For this review, take the finished solid that the model builds, in its own axes (mm). A direction names the side the tool comes from. Round coordinates to 2 decimals unless told otherwise and drop trailing zeros. Use a Markdown table: item, result. Add a question column.
1) Draft analysis for pull direction X (two halves, no side actions). For faces 1 (the face through (6.099, 10, -154)), 2 (the face through (26.101, 10, -154)), 3 (the face through (15.7, 15.2, -313)), 4 (the face through (10, 13.901, -154)), state which applies: pulls with the +X half, pulls with the -X half, needs draft (parallel to the pull), parting line crosses it, or undercut.
2) Consider section A-A (z = -151). Give the number of separate pieces and of enclosed holes in the cut face, plus the area to 3 significant figures.
3) Machinability: for faces 5 (the face through (20, 18.2, -154)), 6 (the face through (20, 20, -154)), which of the approach directions +Z, -Z, +X, -X, +Y, -Y give a long, thin tool a straight path to every point of the face, cutting with its end or side? Answer none if there is none.
4) Wall thickness on line 1 along X through (y, z) = (1.75, -137); line 2 along X through (y, z) = (4, -16); line 3 along Y through (x, z) = (34, -42): over which ranges is each line inside the solid? List them lowest first. Write a range as [from, to].
5) Clearance check with flat-ended pins moving along their axes: P1, Ø3, axis at y = 11.5, z = -233.5, coming from the -X side; P2, Ø4.5, axis at y = 10, z = -198.5, coming from the +X side; P3, Ø2, axis at x = 28.5, z = -165.5, coming from the +Y side. State where each tip first meets the part, or that it passes through.
```python
from build123d import *

# Parameters (mm, degrees)
SKETCH1_R           = 2.1
BOSS_EXTRUDE1_DEPTH = 313


with BuildPart() as part:
    # Sketch1 → Boss-Extrude1 (new body)
    with BuildSketch(Plane.XY):
        Polygon((0, 0), (0, 5.36), (1.8, 7.16), (1.8, 4.500660172), (3.44, 4.500660172), (6.099339828, 7.16), (6.099339828, 12.84), (3.44, 15.499339828), (1.8, 15.499339828), (1.8, 12.84), (0, 14.64), (0, 20), (5.36, 20), (7.16, 18.2), (4.500660172, 18.2), (4.500660172, 16.56), (7.16, 13.900660172), (12.84, 13.900660172), (15.499339828, 16.56), (15.499339828, 18.2), (12.84, 18.2), (14.64, 20), (20, 20), (25.36, 20), (27.16, 18.2), (24.500939946, 18.2), (24.50125838, 16.559689577), (27.161114417, 13.900866058), (32.84111431, 13.901968719), (35.499937829, 16.561824756), (35.49961981, 18.2), (32.84, 18.2), (34.64, 20), (39.999930631, 20), (40.000970647, 14.642698508), (38.201320116, 12.842349107), (38.200803857, 15.501688885), (36.560803888, 15.501370511), (33.901980368, 12.841514474), (33.903083029, 7.161514581), (36.562939066, 4.502691062), (38.202939036, 4.503009436), (38.202422777, 7.162349214), (40.002772178, 5.362698683), (40.003813241, 0), (34.64, 0), (32.84, 1.8), (35.502803549, 1.8), (35.502484821, 3.441825004), (32.842628784, 6.100648523), (27.162628891, 6.099545862), (24.503805372, 3.439689825), (24.504123686, 1.8), (27.16, 1.8), (25.36, 0), (20, 0), (14.64, 0), (12.84, 1.8), (15.499339828, 1.8), (15.499339828, 3.44), (12.84, 6.099339828), (7.16, 6.099339828), (4.500660172, 3.44), (4.500660172, 1.8), (7.16, 1.8), (5.36, 0), align=None)
        with Locations((10, 10)):
            Circle(SKETCH1_R, mode=Mode.SUBTRACT)
        with Locations((30, 10)):
            Circle(SKETCH1_R, mode=Mode.SUBTRACT)
        Polygon((17.300660172, 3.76), (17.300660172, 1.8), (22.700660172, 1.8), (22.700660172, 3.76), (26.100660172, 7.16), (26.100660172, 12.84), (22.699339828, 16.24), (22.699339828, 18.2), (17.300660172, 18.2), (17.300660172, 16.24), (13.900660172, 12.84), (13.900660172, 7.16), align=None, mode=Mode.SUBTRACT)
        Polygon((1.8, 18.2), (3.430660172, 18.2), (3.430660172, 17.63), (2.37, 16.569339828), (1.8, 16.569339828), align=None, mode=Mode.SUBTRACT)
        Polygon((1.8, 3.430660172), (1.8, 1.8), (3.430660172, 1.8), (3.430660172, 2.37), (2.37, 3.430660172), align=None, mode=Mode.SUBTRACT)
        Polygon((38.2, 1.8), (36.569339828, 1.8), (36.569339828, 2.37), (37.63, 3.430660172), (38.2, 3.430660172), align=None, mode=Mode.SUBTRACT)
        Polygon((38.2, 16.569339828), (38.2, 18.2), (36.569339828, 18.2), (36.569339828, 17.63), (37.63, 16.569339828), align=None, mode=Mode.SUBTRACT)
    extrude(amount=-BOSS_EXTRUDE1_DEPTH)


solid = part.part
```
Results list:
| question | item | result |
|---|---|---|
| 1 | face 1 | pulls with the -X half |
| 1 | face 2 | undercut |
| 1 | face 3 | needs draft |
| 1 | face 4 | undercut |
| 2 | separate pieces | 1 |
| 2 | enclosed holes | 7 |
| 2 | area | 292 mm2 |
| 3 | face 5 | +Z, -Z |
| 3 | face 6 | +Z, -Z, +X, -X, +Y |
| 4 | line 1 | [0, 7.11], [12.89, 27.11], [32.89, 40] |
| 4 | line 2 | [0, 5.06], [14.94, 17.06], [22.94, 25.06], [34.94, 40] |
| 4 | line 3 | [0.64, 1.8], [4.94, 7.06], [12.94, 15.06], [18.2, 19.36] |
| 5 | P1 | x = 1.64 |
| 5 | P2 | x = 33.9 |
| 5 | P3 | y = 13.9 |
